```python
from build123d import *

# Parameters (mm, degrees)
BOSS_EXTRUDE1_DEPTH = 14
FILLET1_R           = 1
TAPPED_HOLE1_D      = 4.917


with BuildPart() as part:
    # Sketch1 → Boss-Extrude1 (new body)
    with BuildSketch(Plane(origin=(-7, 0, 0), x_dir=(0, 0, -1), z_dir=(1, 0, 0))):
        Polygon((5.75, -6.3), (-5.75, -6.3), (-7.5, -4.3), (-7.5, -0.8), (-3.9, -0.8), (-3.9, 0), (3.9, 0), (3.9, -0.8), (7.5, -0.8), (7.5, -4.3), align=None)
    extrude(amount=BOSS_EXTRUDE1_DEPTH)

    # Fillet1
    fillet1_edges = [part.edges().sort_by_distance(p)[0] for p in [
        (0, -0.8, -7.5),
        (0, -4.3, -7.5),
        (0, -6.3, -5.75),
        (0, -6.3, 5.75),
        (0, -4.3, 7.5),
        (0, -0.8, 7.5),
    ]]
    fillet(fillet1_edges, radius=FILLET1_R)

    # Tapped Hole1 (through all)
    with Locations(Plane(origin=(0, 0, 0), x_dir=(1, 0, 0), z_dir=(0, 1, 0))):
        with Locations((0, 0)):
            Hole(TAPPED_HOLE1_D / 2)


solid = part.part
```
Verification items for the finished model (mm, model axes). A direction names the side the tool comes from. Round coordinates to 2 decimals unless told otherwise and drop trailing zeros. Order: outer loops, then holes, each group sorted by start corner. A loop starts at its lowest first (then second) coordinate and runs counter-clockwise, first axis right, second up. Notation, with made-up numbers: (-30.5, 0) - (28.5, 0) arc R20 ccw to (28.5, 9) - close; hole circle Ø7 at (14, 70.25). An arc over 180 degrees is marked (long way). Use CSV: the item, a comma, the result in double quotes. Start each with the question number.
1) Section check C-C, the plane y = -2.75. Record the cut outline in (x, z).
2) Section check B-B, the plane z = 0. Record the cut outline in (x, y), plus the area to 3 significant figures.
3) Section check A-A, the plane x = 0. Record the cut outline in (y, z).
4) Mould release check, pull along X, two halves, no side actions. Record for faces 4 (the flat face through (-7, -3, 0)), 5 (the flat face through (0, -3, 7.5)), 6 (the cylindrical face through (-2.345, -3.194, -0.738)): +X half, -X half, draft (parallel to the pull), parting line (faces both ways), or undercut.
5) Go/stop test with flat-tipped pins: P1, Ø3, axis at x = -3, z = -5.5, coming from the +Y side; P2, Ø4.5, axis at x = 0, z = 0, coming from the +Y side. Record where each tip stops, or that it passes through.
6) Access from +Z, -Z, +X, -X, +Y, -Y to the whole of each face (thin tool, end or side, straight path). Record for faces 1 (the flat face through (0, -0.8, 5)), 2 (the flat face through (0, 0, 3)), 3 (the flat face through (0, -0.8, -5)).
7) Thickness scan on L1, parallel to Z at x = 0, y = -3; L2, parallel to Y at x = 0.5, z = -5.25; L3, parallel to Z at x = 0, y = -4.5. Record the ranges inside material, lowest first.
8) Section check D-D, the plane x = 6.25. Record the cut outline in (y, z), plus the area to 3 significant figures.
Answers:
1,outline,"(-7, -7.5) - (7, -7.5) - (7, 7.5) - (-7, 7.5) - close; hole circle Ø4.92 at (0, 0)"
2,outline,"(-7, -6.3) - (-2.46, -6.3) - (-2.46, 0) - (-7, 0) - close; (2.46, -6.3) - (7, -6.3) - (7, 0) - (2.46, 0) - close"
2,area,"57.2 mm²"
3,outline,"(-6.3, -5.3) arc R1 ccw to (-5.96, -6.05) - (-4.58, -7.25) arc R1 ccw to (-3.92, -7.5) - (-1.8, -7.5) arc R1 ccw to (-0.8, -6.5) - (-0.8, -3.9) - (0, -3.9) - (0, -2.46) - (-6.3, -2.46) - close; (-6.3, 2.46) - (0, 2.46) - (0, 3.9) - (-0.8, 3.9) - (-0.8, 6.5) arc R1 ccw to (-1.8, 7.5) - (-3.92, 7.5) arc R1 ccw to (-4.58, 7.25) - (-5.96, 6.05) arc R1 ccw to (-6.3, 5.3) - close"
4,face 4,"-X half"
4,face 5,"draft"
4,face 6,"undercut"
5,P1,"stops at y = -0.8"
5,P2,"passes through"
6,face 1,"+Z, +X, -X, +Y"
6,face 2,"+Z, -Z, +X, -X, +Y"
6,face 3,"-Z, +X, -X, +Y"
7,L1,"z = -7.5 to -2.46, 2.46 to 7.5"
7,L2,"y = -6.3 to -0.8"
7,L3,"z = -7.32 to -2.46, 2.46 to 7.32"
8,outline,"(-6.3, -5.3) arc R1 ccw to (-5.96, -6.05) - (-4.58, -7.25) arc R1 ccw to (-3.92, -7.5) - (-1.8, -7.5) arc R1 ccw to (-0.8, -6.5) - (-0.8, -3.9) - (0, -3.9) - (0, 3.9) - (-0.8, 3.9) - (-0.8, 6.5) arc R1 ccw to (-1.8, 7.5) - (-3.92, 7.5) arc R1 ccw to (-4.58, 7.25) - (-5.96, 6.05) arc R1 ccw to (-6.3, 5.3) - close"
8,area,"84.7 mm²"
